Input: part model. Units: mm. Frame: model coordinates. Coordinates: 2 decimals unless noted, no trailing zeros. Write each loop counter-clockwise with the first axis right and the second up, starting at its lowest first coordinate (ties: lowest second). Pieces come first, ordered by that corner, then holes. Notation, with made-up numbers: M 3.5,-28.5 L 21.5,-28.5 A33 ccw 21.5,1.5 Z; hole C 26,89.5 d10. An arc over 180 degrees is marked long. Write each question's results on one line, items separated by ' | '. Start each with the question number.
1. Section query D-D, the plane z = -72.5. Output: boundary loops of the cut face in (x, y), and give its area (3 significant figures).
2. Section query A-A, the plane z = -97.5. Output: boundary loops of the cut face in (x, y).
3. Ray query, probe 1 along X at (y, z) = (-5, 72.5); probe 2 along X at (y, z) = (-7, -41.11); probe 3 along X at (y, z) = (-6.5, 3). Return the intervals inside material, ascending.
4. Section query C-C, the plane y = -2. Count the separate pieces of the cut face and the enclosed holes in it, and give its area (3 significant figures).
5. Section query B-B, the plane z = -9.86. Output: boundary loops of the cut face in (x, y), and give its area (3 significant figures).
6. First-contact query: pin 1 (6.5 mm diameter, centred on x = -25, z = -97.5, fed in from +Y). Flat tip, straight axial feed; report the tip coordinate or a pass-through.
```python
from build123d import *

# Parameters (mm, degrees)
SKETCH2_W                  = 80
SKETCH2_H                  = 225
BOSS_EXTRUDE1_DEPTH        = 10
CUT_EXTRUDE1_REACH         = 121.818
SKETCH3_R                  = 8
M8_CLEARANCE_HOLE1_D       = 8.4
F_8_0MM_DOWEL_HOLE1_D      = 8
F_10_0_10_DIAMETER_HOLE1_D = 10
M6_CLEARANCE_HOLE1_D       = 6.4
CUT_EXTRUDE2_REACH         = 121.818
SKETCH16_R                 = 7


with BuildPart() as part:
    # Sketch2 → Boss-Extrude1 (new body)
    with BuildSketch(Plane(origin=(0, 0, 0), x_dir=(1, 0, 0), z_dir=(0, 1, 0))):
        Rectangle(SKETCH2_W, SKETCH2_H)
    extrude(amount=-BOSS_EXTRUDE1_DEPTH)

    # Sketch3 → Cut-Extrude1 (cut, up to next)
    with BuildSketch(Plane(origin=(0, 0, 0), x_dir=(1, 0, 0), z_dir=(0, 1, 0)), mode=Mode.PRIVATE) as cut_extrude1_sk1:
        with Locations(Location((15, -7, 0), (0, 0, 270))):
            Circle(SKETCH3_R)
    cut_extrude1_tool1 = extrude(cut_extrude1_sk1.sketch, amount=-CUT_EXTRUDE1_REACH, mode=Mode.PRIVATE) & part.part
    # Sketch3 → Cut-Extrude1 (cut, up to next)
    with BuildSketch(Plane(origin=(0, 0, 0), x_dir=(1, 0, 0), z_dir=(0, 1, 0)), mode=Mode.PRIVATE) as cut_extrude1_sk2:
        with Locations(Location((15, 41.11, 0), (0, 0, 270))):
            Circle(SKETCH3_R)
    cut_extrude1_tool2 = extrude(cut_extrude1_sk2.sketch, amount=-CUT_EXTRUDE1_REACH, mode=Mode.PRIVATE) & part.part
    # Sketch3 → Cut-Extrude1 (cut, up to next)
    with BuildSketch(Plane(origin=(0, 0, 0), x_dir=(1, 0, 0), z_dir=(0, 1, 0)), mode=Mode.PRIVATE) as cut_extrude1_sk3:
        with Locations(Location((15, -72.5, 0), (0, 0, 270))):
            Circle(SKETCH3_R)
    cut_extrude1_tool3 = extrude(cut_extrude1_sk3.sketch, amount=-CUT_EXTRUDE1_REACH, mode=Mode.PRIVATE) & part.part
    # Sketch3 → Cut-Extrude1 (cut, up to next)
    with BuildSketch(Plane(origin=(0, 0, 0), x_dir=(1, 0, 0), z_dir=(0, 1, 0)), mode=Mode.PRIVATE) as cut_extrude1_sk4:
        with Locations(Location((-20, -72.5, 0), (0, 0, 270))):
            Circle(SKETCH3_R)
    cut_extrude1_tool4 = extrude(cut_extrude1_sk4.sketch, amount=-CUT_EXTRUDE1_REACH, mode=Mode.PRIVATE) & part.part
    # Sketch3 → Cut-Extrude1 (cut, up to next)
    with BuildSketch(Plane(origin=(0, 0, 0), x_dir=(1, 0, 0), z_dir=(0, 1, 0)), mode=Mode.PRIVATE) as cut_extrude1_sk5:
        with Locations(Location((-20, -7, 0), (0, 0, 270))):
            Circle(SKETCH3_R)
    cut_extrude1_tool5 = extrude(cut_extrude1_sk5.sketch, amount=-CUT_EXTRUDE1_REACH, mode=Mode.PRIVATE) & part.part
    # Sketch3 → Cut-Extrude1 (cut, up to next)
    with BuildSketch(Plane(origin=(0, 0, 0), x_dir=(1, 0, 0), z_dir=(0, 1, 0)), mode=Mode.PRIVATE) as cut_extrude1_sk6:
        with Locations(Location((-20, 41.11, 0), (0, 0, 270))):
            Circle(SKETCH3_R)
    cut_extrude1_tool6 = extrude(cut_extrude1_sk6.sketch, amount=-CUT_EXTRUDE1_REACH, mode=Mode.PRIVATE) & part.part
    # Sketch3 → Cut-Extrude1 (cut, up to next)
    with BuildSketch(Plane(origin=(0, 0, 0), x_dir=(1, 0, 0), z_dir=(0, 1, 0)), mode=Mode.PRIVATE) as cut_extrude1_sk7:
        with Locations(Location((-20, 72.5, 0), (0, 0, 270))):
            Circle(SKETCH3_R)
    cut_extrude1_tool7 = extrude(cut_extrude1_sk7.sketch, amount=-CUT_EXTRUDE1_REACH, mode=Mode.PRIVATE) & part.part
    # Sketch3 → Cut-Extrude1 (cut, up to next)
    with BuildSketch(Plane(origin=(0, 0, 0), x_dir=(1, 0, 0), z_dir=(0, 1, 0)), mode=Mode.PRIVATE) as cut_extrude1_sk8:
        with Locations(Location((15, 72.5, 0), (0, 0, 270))):
            Circle(SKETCH3_R)
    cut_extrude1_tool8 = extrude(cut_extrude1_sk8.sketch, amount=-CUT_EXTRUDE1_REACH, mode=Mode.PRIVATE) & part.part
    add(cut_extrude1_tool1.solids().sort_by_distance((15, 0, 7))[0], mode=Mode.SUBTRACT)
    add(cut_extrude1_tool2.solids().sort_by_distance((15, 0, -41.11))[0], mode=Mode.SUBTRACT)
    add(cut_extrude1_tool3.solids().sort_by_distance((15, 0, 72.5))[0], mode=Mode.SUBTRACT)
    add(cut_extrude1_tool4.solids().sort_by_distance((-20, 0, 72.5))[0], mode=Mode.SUBTRACT)
    add(cut_extrude1_tool5.solids().sort_by_distance((-20, 0, 7))[0], mode=Mode.SUBTRACT)
    add(cut_extrude1_tool6.solids().sort_by_distance((-20, 0, -41.11))[0], mode=Mode.SUBTRACT)
    add(cut_extrude1_tool7.solids().sort_by_distance((-20, 0, -72.5))[0], mode=Mode.SUBTRACT)
    add(cut_extrude1_tool8.solids().sort_by_distance((15, 0, -72.5))[0], mode=Mode.SUBTRACT)

    # M8 Clearance Hole1 (through all)
    with Locations(Plane(origin=(0, 0, 0), x_dir=(1, 0, 0), z_dir=(0, 1, 0))):
        with Locations((-25, -97.5), (15, -97.5), (15, 97.5), (-25, 97.5)):
            Hole(M8_CLEARANCE_HOLE1_D / 2)

    # 8.0mm Dowel Hole1 (through all)
    with Locations(Plane(origin=(0, 0, 0), x_dir=(1, 0, 0), z_dir=(0, 1, 0))):
        with Locations((-5, 97.5), (-5, -97.5)):
            Hole(F_8_0MM_DOWEL_HOLE1_D / 2)

    # 10.0 _10_ Diameter Hole1 (through all)
    with Locations(Plane(origin=(0, 0, 0), x_dir=(1, 0, 0), z_dir=(0, 1, 0))):
        with Locations((-2.5, -72.5), (-2.5, 72.5), (20, 22), (-25, -36)):
            Hole(F_10_0_10_DIAMETER_HOLE1_D / 2)

    # M6 Clearance Hole1 (through all)
    with Locations(Plane(origin=(0, 0, 0), x_dir=(1, 0, 0), z_dir=(0, 1, 0))):
        with Locations((24, -34.64), (-1, -34.64)):
            Hole(M6_CLEARANCE_HOLE1_D / 2)

    # Sketch16 → Cut-Extrude2 (cut, up to next)
    with BuildSketch(Plane(origin=(0, 0, 0), x_dir=(1, 0, 0), z_dir=(0, 1, 0)), mode=Mode.PRIVATE) as cut_extrude2_sk1:
        with Locations(Location((11.5, 9.86, 0), (0, 0, 270))):
            Circle(SKETCH16_R)
    cut_extrude2_tool1 = extrude(cut_extrude2_sk1.sketch, amount=-CUT_EXTRUDE2_REACH, mode=Mode.PRIVATE) & part.part
    add(cut_extrude2_tool1.solids().sort_by_distance((11.5, 0, -9.86))[0], mode=Mode.SUBTRACT)


solid = part.part
```
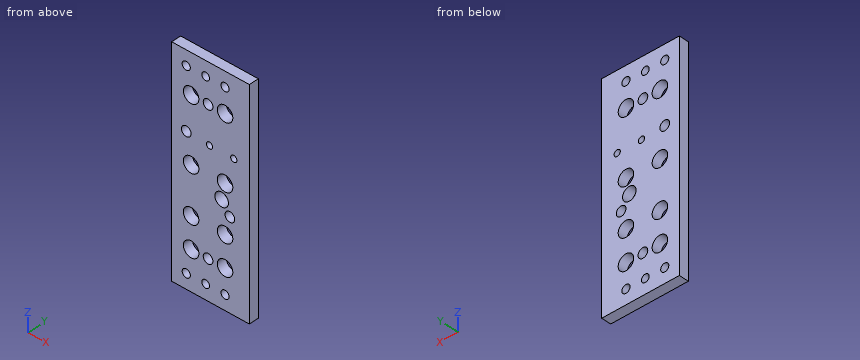
Answer:
1) outline: M -40,-10 L -28,-10 L -28,0 L -40,0 Z; M -12,-10 L -7.5,-10 L -7.5,0 L -12,0 Z; M 2.5,-10 L 7,-10 L 7,0 L 2.5,0 Z; M 23,-10 L 40,-10 L 40,0 L 23,0 Z | area: 380 mm^2
2) outline: M -40,-10 L -29.2,-10 L -29.2,0 L -40,0 Z; M -20.8,-10 L -9,-10 L -9,0 L -20.8,0 Z; M -1,-10 L 10.8,-10 L 10.8,0 L -1,0 Z; M 19.2,-10 L 40,-10 L 40,0 L 19.2,0 Z
3) probe 1: -40 to -28, -12 to -7.5, 2.5 to 7, 23 to 40 | probe 2: -40 to -28, -12 to 7, 23 to 40 | probe 3: -40 to -26.93, -13.07 to 8.07, 21.93 to 40
4) separate pieces: 1 | enclosed holes: 21 | area: 15,500 mm^2
5) outline: M -40,-10 L 4.5,-10 L 4.5,0 L -40,0 Z; M 18.5,-10 L 40,-10 L 40,0 L 18.5,0 Z | area: 660 mm^2
6) pin 1: through
